```python
from build123d import *

# Parameters (mm, degrees)
SKETCH1_W           = 18
SKETCH1_H           = 18
BOSS_EXTRUDE1_DEPTH = 5
SKETCH4_W           = 12
SKETCH4_H           = 12
CUT_EXTRUDE1_DEPTH  = 3
SKETCH5_W           = 18
SKETCH5_H           = 11
BOSS_EXTRUDE2_DEPTH = 11
CUT_EXTRUDE2_DEPTH  = 15.5


with BuildPart() as part:
    # Sketch1 → Boss-Extrude1 (new body)
    with BuildSketch(Plane(origin=(0, 0, 0), x_dir=(1, 0, 0), z_dir=(0, 1, 0))):
        with Locations((-259.2, 371.7)):
            Rectangle(SKETCH1_W, SKETCH1_H)
    extrude(amount=BOSS_EXTRUDE1_DEPTH)

    # Sketch4 → Cut-Extrude1 (cut)
    with BuildSketch(Plane.XZ):
        with Locations((-259.2, -371.7)):
            Rectangle(SKETCH4_W, SKETCH4_H)
    extrude(amount=-CUT_EXTRUDE1_DEPTH, mode=Mode.SUBTRACT)

    # Sketch5 → Boss-Extrude2 (add)
    with BuildSketch(Plane(origin=(0, 5, 0), x_dir=(1, 0, 0), z_dir=(0, 1, 0))):
        with Locations((-259.2, 371.7)):
            Rectangle(SKETCH5_W, SKETCH5_H)
    extrude(amount=BOSS_EXTRUDE2_DEPTH)

    # Sketch7 → Cut-Extrude2 (cut, through all)
    with BuildSketch(Plane.XY.offset(-366.2)):
        with BuildLine():
            ThreePointArc((-261.2, 8.5), (-259.2, 6.5), (-257.2, 8.5))
            Line((-257.2, 8.5), (-261.2, 8.5))
        make_face()
        with BuildLine():
            Line((-261.2, 8.5), (-257.2, 8.5))
            ThreePointArc((-257.2, 8.5), (-259.2, 10.5), (-261.2, 8.5))
        make_face()
        with BuildLine():
            Line((-257.2, 16), (-259.2, 16))
            Line((-259.2, 16), (-261.2, 16))
            Line((-261.2, 16), (-261.2, 8.5))
            ThreePointArc((-261.2, 8.5), (-259.2, 10.5), (-257.2, 8.5))
            Line((-257.2, 8.5), (-257.2, 16))
        make_face()
        Polygon((-250.2, 16), (-254.2, 16), (-250.2, 12), align=None)
        Polygon((-268.2, 12), (-264.2, 16), (-268.2, 16), align=None)
    extrude(amount=-CUT_EXTRUDE2_DEPTH, mode=Mode.SUBTRACT)


solid = part.part
```
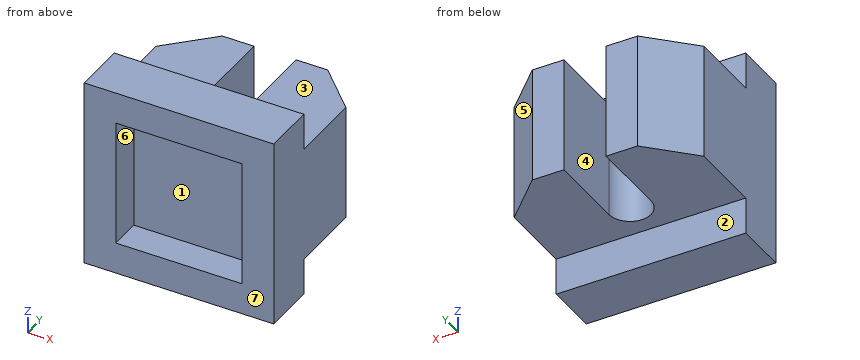
Can you work these out from the model? Positions are in its coordinate system, mm. Face numbers are marked on the shaded views. A direction names the side the tool comes from. Round coordinates to 2 decimals unless told otherwise and drop trailing zeros. Order: outer loops, then holes, each group sorted by start corner. A loop starts at its lowest first (then second) coordinate and runs counter-clockwise, first axis right, second up.
(1) If we section it at D-D (y = 8): Please give me the cut outline in (x, z), plus the area to 3 significant figures.
Results are:
outline: (-268.2, -377.2) - (-261.14, -377.2) - (-261.14, -366.2) - (-268.2, -366.2) - close; (-257.26, -377.2) - (-250.2, -377.2) - (-250.2, -366.2) - (-257.26, -366.2) - close
area: 155 mm2
(2) If I drill on L1, parallel to X at y = 1.5, z = -367.5; L2, parallel to Y at x = -261.5, z = -372; L3, parallel to X at y = 10, z = -377, over which ranges is the centre line in solid material (lowest first)?
Results are:
L1: x = -268.2 to -265.2, -253.2 to -250.2
L2: y = 3 to 16
L3: x = -268.2 to -261.2, -257.2 to -250.2
(3) If we section it at A-A (y = 2.5): Please give me the cut outline in (x, z).
Results are:
outline: (-268.2, -380.7) - (-250.2, -380.7) - (-250.2, -362.7) - (-268.2, -362.7) - close; hole (-265.2, -377.7) - (-253.2, -377.7) - (-253.2, -365.7) - (-265.2, -365.7) - close
(4) We'd pull the mould along X, two halves only. Please class the marked faces 5, 6 and 7: +X half, -X half, draft (parallel to the pull), parting line (faces both ways), or undercut.
Results are:
face 5: +X half
face 6: undercut
face 7: draft
(5) If we section it at B-B (x = -251.5): Please give me the cut outline in (y, z).
Results are:
outline: (0, -380.7) - (5, -380.7) - (5, -377.2) - (13.3, -377.2) - (13.3, -366.2) - (5, -366.2) - (5, -362.7) - (0, -362.7) - close
(6) If we section it at C-C (z = -368.5): Please give me the cut outline in (x, y).
Results are:
outline: (-268.2, 0) - (-265.2, 0) - (-265.2, 3) - (-253.2, 3) - (-253.2, 0) - (-250.2, 0) - (-250.2, 12) - (-254.2, 16) - (-257.2, 16) - (-257.2, 8.5) arc R2 cw to (-261.2, 8.5) - (-261.2, 16) - (-264.2, 16) - (-268.2, 12) - close
(7) On a 3-axis mill with a long thin cutter (end or side, diameter ignored), from which of +Z, -Z, +X, -X, +Y, -Y can I reach the whole of each face in a straight line? I mean the marked faces 1, 2, 3 and 4. Say none if no direction works.
Results are:
face 1: -Y
face 2: -Z, +X, -X, +Y
face 3: +Z, +X, -X, +Y
face 4: +Z, -Z, +Y
(8) I'm going to push flat-ended pins straight in: pin 1 (3 mm diameter, centred on x = -255.5, z = -379, fed in from +Y); pin 2 (6 mm diameter, centred on x = -258.5, z = -374, fed in from -Y); pin 3 (1 mm diameter, centred on x = -264.5, z = -378.5, fed in from -Y); pin 4 (3.5 mm diameter, centred on x = -255.5, y = 10.5, fed in from -Z). Where does each tip first touch, or does it pass through?
Results are:
pin 1: stops at y = 5
pin 2: stops at y = 3
pin 3: stops at y = 0
pin 4: stops at z = -377.2
